The listing builds one solid part. Answer for the finished solid, in the listing's coordinates (mm). Face numbers are marked on the shaded views. Give positions to 0.01 mm unless a question says otherwise; leave off trailing zeros. Order: outer loops, then holes, each group sorted by start corner. A loop starts at its lowest first (then second) coordinate and runs counter-clockwise, first axis right, second up. Notation, with made-up numbers: (-15, 31.25) - (15, 31.25) arc R15 ccw to (15, 48.25) - close; hole circle Ø6 at (87.5, 9.5). An arc over 180 degrees is marked (long way). Answer in a Markdown table with one row per item. Add a question column.
```python
from build123d import *

# Parameters (mm, degrees)
SKETCH2_W            = 444.5
SKETCH2_H            = 584.2
BOSS_EXTRUDE1_DEPTH  = 6.35
MOVE_START           = -2.17182791
MOVE_FACE1_OUTLINE_W = 448
MOVE_FACE1_OUTLINE_H = 9
MOVE_FACE1_DEPTH     = 2.17182791
CONVERT_SOLID1_START = -222.25
CONVERT_SOLID1_DEPTH = 444.5
SKETCH7_W            = 19.05
SKETCH7_H            = 5.08
CUT_EXTRUDE1_DEPTH   = 626.080014878
SKETCH9_R            = 1.905
CUT_EXTRUDE2_DEPTH   = 1.2192
CHAMFER1_SIZE        = 2.54


# Read off the part's stored shape, not the designer's step: Move Face1, Convert-Solid1
with BuildPart() as part:
    # Sketch2 → Boss-Extrude1 (new body)
    with BuildSketch(Plane(origin=(0, 0, 0), x_dir=(1, 0, 0), z_dir=(0, 1, 0))):
        with Locations((0, 292.1)):
            Rectangle(SKETCH2_W, SKETCH2_H)
    extrude(amount=-BOSS_EXTRUDE1_DEPTH)

    # Move Face1 outline → Move Face1 (cut)
    with BuildSketch(Plane(origin=(0, 0, 0), x_dir=(1, 0, 0), z_dir=(0, 0.3420201433256691, -0.9396926207859083)).offset(MOVE_START)):
        with Locations((0, 3.5)):
            Rectangle(MOVE_FACE1_OUTLINE_W, MOVE_FACE1_OUTLINE_H)
    extrude(amount=MOVE_FACE1_DEPTH, mode=Mode.SUBTRACT)

    # Convert-Solid1 outline → Convert-Solid1 (cut)
    with BuildSketch(Plane.YZ.offset(CONVERT_SOLID1_START)):
        with BuildLine():
            Line((-6.037256781, -3.17046592), (-6.35, -2.311210988))
            Line((-6.35, -2.311210988), (-6.35, -583.2856))
            Line((-6.35, -583.2856), (-1.6764, -583.2856))
            ThreePointArc((-1.6764, -583.2856), (-1.137584633, -583.062415367), (-0.9144, -582.5236))
            Line((-0.9144, -582.5236), (-0.9144, -2.394147319))
            ThreePointArc((-0.9144, -2.394147319), (-1.239334756, -1.769953461), (-1.937019349, -1.678101541))
            Line((-1.937019349, -1.678101541), (-6.037256781, -3.17046592))
        make_face()
        with BuildLine():
            Line((0, 0), (-2.249762568, -0.818846609))
            ThreePointArc((-2.249762568, -0.818846609), (-0.714856462, -1.020920831), (0, -2.394147319))
            Line((0, -2.394147319), (0, 0))
        make_face()
        with BuildLine():
            Line((0, -584.2), (0, -582.5236))
            ThreePointArc((0, -582.5236), (-0.491006192, -583.708993808), (-1.6764, -584.2))
            Line((-1.6764, -584.2), (0, -584.2))
        make_face()
    extrude(amount=CONVERT_SOLID1_DEPTH, mode=Mode.SUBTRACT)

    # Sketch7 → Cut-Extrude1 (cut, through all)
    with BuildSketch(Plane(origin=(0, 0, 0), x_dir=(1, 0, 0), z_dir=(0, 1, 0))):
        with Locations((-212.725, 2.54)):
            Rectangle(SKETCH7_W, SKETCH7_H)
        with Locations((212.725, 2.54)):
            Rectangle(SKETCH7_W, SKETCH7_H)
    extrude(amount=-CUT_EXTRUDE1_DEPTH, mode=Mode.SUBTRACT)

    # Sketch9 → Cut-Extrude2 (cut)
    with BuildSketch(Plane(origin=(0, 0, 0), x_dir=(1, 0, 0), z_dir=(0, 1, 0))):
        with Locations(Location((-210.82, 25.4, 0), (0, 0, 270))):
            Circle(SKETCH9_R)
        with Locations(Location((-210.82, 317.5, 0), (0, 0, 270))):
            Circle(SKETCH9_R)
        with Locations(Location((-210.82, 558.8, 0), (0, 0, 270))):
            Circle(SKETCH9_R)
        with Locations(Location((210.82, 558.8, 0), (0, 0, 90))):
            Circle(SKETCH9_R)
        with Locations(Location((210.82, 317.5, 0), (0, 0, 90))):
            Circle(SKETCH9_R)
        with Locations(Location((210.82, 25.4, 0), (0, 0, 90))):
            Circle(SKETCH9_R)
        with Locations(Location((-44.0182, 167.64, 0), (0, 0, 90))):
            Circle(SKETCH9_R)
        with Locations(Location((-44.0182, 467.36, 0), (0, 0, 270))):
            Circle(SKETCH9_R)
        with Locations(Location((44.0182, 467.36, 0), (0, 0, 90))):
            Circle(SKETCH9_R)
        with Locations(Location((44.0182, 167.64, 0), (0, 0, 270))):
            Circle(SKETCH9_R)
    extrude(amount=-CUT_EXTRUDE2_DEPTH, mode=Mode.SUBTRACT)

    # Chamfer1
    chamfer1_edges = [part.edges().sort_by_distance(p)[0] for p in [
        (-222.25, -6.35, -583.7428),
        (222.25, -6.35, -583.7428),
        (-222.25, -0.4572, -5.08),
        (-203.2, -6.193628391, -2.740838454),
        (222.25, -0.4572, -5.08),
        (203.2, -6.193628391, -2.740838454),
    ]]
    chamfer(chamfer1_edges, length=CHAMFER1_SIZE)


solid = part.part
```
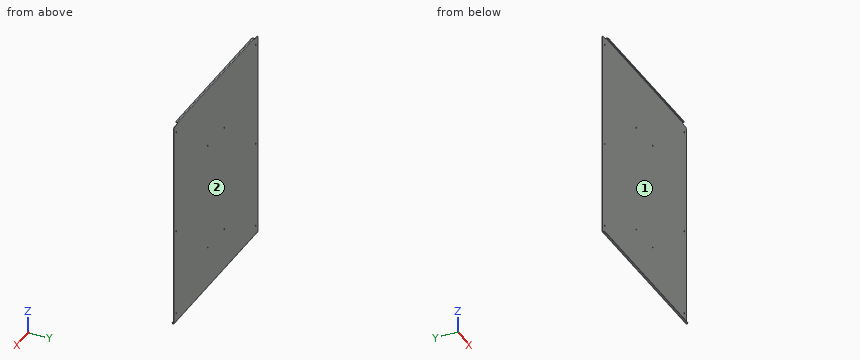
(1) Straight lines are drawn through the part: line 1 (X direction, y = -0.4, z = -467.36); line 2 (X direction, y = -0.25, z = -558.8) (3 decimals); line 3 (Z direction, x = 199.5, y = -2.5). For each, find the intervals that lie inside material, in ascending order.
(2) Find section B-B, the plane z = -61. Write down the section's boundary in (x, y).
(3) The mould has two halves that part along Z. Classify the marked faces 1 and 2: +Z half, -Z half, draft (parallel to the pull), parting line (faces both ways), or undercut.
(4) Each of these flat-tipped pins is pushed along its axis until it touches: P1, Ø1, axis at x = 209.5, y = -0.5, coming from the +Z side; P2, Ø2, axis at y = -3.5, z = -128.5, coming from the -X side; P3, Ø12, axis at x = 163.5, z = -274.5, coming from the -Y side; P4, Ø3, axis at y = -1.5, z = -3.5, coming from the -X side. Where does it stop, or does it pass through?
(5) Find section A-A, the plane x = -69.5. Write down the section's boundary in (y, z), plus the area to 3 significant figures.
Answer key:
| question | item | result |
|---|---|---|
| 1 | line 1 | -222.25 to -45.92, -42.11 to 42.11, 45.92 to 222.25 |
| 1 | line 2 | -222.25 to -212.725, -208.915 to 208.915, 212.725 to 222.25 |
| 1 | line 3 | -584.2 to -583.29, -1.88 to -0.91 |
| 2 | outline | (-222.25, -0.91) - (222.25, -0.91) - (222.25, 0) - (-222.25, 0) - close |
| 3 | face 1 | undercut |
| 3 | face 2 | draft |
| 4 | P1 | z = -5.08 |
| 4 | P2 | through |
| 4 | P3 | y = -0.91 |
| 4 | P4 | x = -203.2 |
| 5 | outline | (-6.35, -584.2) - (-1.68, -584.2) arc R1.68 ccw to (0, -582.52) - (0, -2.39) arc R1.68 ccw to (-2.25, -0.82) - (-6.35, -2.31) - (-6.04, -3.17) - (-1.94, -1.68) arc R0.76 cw to (-0.91, -2.39) - (-0.91, -582.52) arc R0.76 cw to (-1.68, -583.29) - (-6.35, -583.29) - close |
| 5 | area | 543 mm² |
